from build123d import *

# Parameters (mm, degrees)
SKETCH1_R           = 2.1
SKETCH1_R_2         = 2.55
SKETCH1_R_3         = 2.54
BOSS_EXTRUDE1_DEPTH = 4


with BuildPart() as part:
    # Sketch1 → Boss-Extrude1 (new body)
    with BuildSketch(Plane(origin=(0, 0, 0), x_dir=(-1, 0, 0), z_dir=(0, 0, -1))):
        with BuildLine():
            Line((87.42535625, -29.106339063), (52.57464375, -20.393660937))
            ThreePointArc((52.57464375, -20.393660937), (47.11794562, -16.84635803), (45, -10.692235936))
            Line((45, -10.692235936), (45, -8))
            ThreePointArc((45, -8), (44.853553391, -7.646446609), (44.5, -7.5))
            Line((44.5, -7.5), (38, -7.5))
            ThreePointArc((38, -7.5), (37.646446609, -7.353553391), (37.5, -7))
            Line((37.5, -7), (37.5, 3))
            ThreePointArc((37.5, 3), (37.646446609, 3.353553391), (38, 3.5))
            Line((38, 3.5), (39.5, 3.5))
            ThreePointArc((39.5, 3.5), (39.853553391, 3.353553391), (40, 3))
            Line((40, 3), (40, -4.5))
            ThreePointArc((40, -4.5), (40.146446609, -4.853553391), (40.5, -5))
            Line((40.5, -5), (44.5, -5))
            ThreePointArc((44.5, -5), (44.853553391, -4.853553391), (45, -4.5))
            Line((45, -4.5), (45, 38.692235936))
            ThreePointArc((45, 38.692235936), (47.11794562, 44.84635803), (52.57464375, 48.393660937))
            Line((52.57464375, 48.393660937), (87.42535625, 57.106339063))
            ThreePointArc((87.42535625, 57.106339063), (92.88205438, 60.65364197), (95, 66.807764064))
            Line((95, 66.807764064), (95, 85))
            ThreePointArc((95, 85), (92.071067812, 92.071067812), (85, 95))
            Line((85, 95), (80.600023778, 95))
            ThreePointArc((80.600023778, 95), (75.38177505, 94.307249421), (70.525020806, 92.276988022))
            ThreePointArc((70.525020806, 92.276988022), (0, 73.215904175), (-70.525020806, 92.276988022))
            ThreePointArc((-70.525020806, 92.276988022), (-75.38177505, 94.307249421), (-80.600023778, 95))
            Line((-80.600023778, 95), (-85, 95))
            ThreePointArc((-85, 95), (-92.071067812, 92.071067812), (-95, 85))
            Line((-95, 85), (-95, 57.30993956))
            ThreePointArc((-95, 57.30993956), (-93.292887614, 51.721736358), (-88.754396995, 48.041471336))
            Line((-88.754396995, 48.041471336), (-51.245603005, 32.847708996))
            ThreePointArc((-51.245603005, 32.847708996), (-46.707112386, 29.167443975), (-45, 23.579240773))
            Line((-45, 23.579240773), (-45, -4.5))
            ThreePointArc((-45, -4.5), (-44.853553391, -4.853553391), (-44.5, -5))
            Line((-44.5, -5), (-40.5, -5))
            ThreePointArc((-40.5, -5), (-40.146446609, -4.853553391), (-40, -4.5))
            Line((-40, -4.5), (-40, 3))
            ThreePointArc((-40, 3), (-39.853553391, 3.353553391), (-39.5, 3.5))
            Line((-39.5, 3.5), (-38, 3.5))
            ThreePointArc((-38, 3.5), (-37.646446609, 3.353553391), (-37.5, 3))
            Line((-37.5, 3), (-37.5, -7))
            ThreePointArc((-37.5, -7), (-37.646446609, -7.353553391), (-38, -7.5))
            Line((-38, -7.5), (-44.5, -7.5))
            ThreePointArc((-44.5, -7.5), (-44.853553391, -7.646446609), (-45, -8))
            Line((-45, -8), (-45, -23.579240773))
            ThreePointArc((-45, -23.579240773), (-46.707112386, -29.167443975), (-51.245603005, -32.847708996))
            Line((-51.245603005, -32.847708996), (-88.754396995, -48.041471336))
            ThreePointArc((-88.754396995, -48.041471336), (-93.292887614, -51.721736358), (-95, -57.30993956))
            Line((-95, -57.30993956), (-95, -85))
            ThreePointArc((-95, -85), (-92.071067812, -92.071067812), (-85, -95))
            Line((-85, -95), (-80.600023778, -95))
            ThreePointArc((-80.600023778, -95), (-75.38177505, -94.307249421), (-70.525020806, -92.276988022))
            ThreePointArc((-70.525020806, -92.276988022), (0, -73.215904175), (70.525020806, -92.276988022))
            ThreePointArc((70.525020806, -92.276988022), (75.38177505, -94.307249421), (80.600023778, -95))
            Line((80.600023778, -95), (85, -95))
            ThreePointArc((85, -95), (92.071067812, -92.071067812), (95, -85))
            Line((95, -85), (95, -38.807764064))
            ThreePointArc((95, -38.807764064), (92.88205438, -32.65364197), (87.42535625, -29.106339063))
        make_face()
        with Locations(Location((-85, -85, 0), (0, 0, 180))):
            Circle(SKETCH1_R, mode=Mode.SUBTRACT)
        with Locations(Location((-85, 85, 0), (0, 0, 180))):
            Circle(SKETCH1_R, mode=Mode.SUBTRACT)
        with Locations(Location((85, 85, 0), (0, 0, 180))):
            Circle(SKETCH1_R, mode=Mode.SUBTRACT)
        with Locations(Location((85, -85, 0), (0, 0, 180))):
            Circle(SKETCH1_R, mode=Mode.SUBTRACT)
        with Locations(Location((25, 17.873209062, 0), (0, 0, 180))):
            Circle(SKETCH1_R_2, mode=Mode.SUBTRACT)
        with Locations(Location((25, -26.606790938, 0), (0, 0, 180))):
            Circle(SKETCH1_R_3, mode=Mode.SUBTRACT)
        with Locations(Location((-25, -26.606790938, 0), (0, 0, 180))):
            Circle(SKETCH1_R_3, mode=Mode.SUBTRACT)
        with Locations(Location((-25, 17.873209062, 0), (0, 0, 180))):
            Circle(SKETCH1_R_2, mode=Mode.SUBTRACT)
    extrude(amount=-BOSS_EXTRUDE1_DEPTH)


solid = part.part
Model file for the job. Use its own axes, mm. A direction names the side the tool comes from. Give positions to 0.01 mm unless a question says otherwise; leave off trailing zeros. Loops run counter-clockwise (first coordinate to the right, second up) from the corner with the lowest first, then second, coordinate; pieces in that order, holes last. Notation, with made-up numbers: (64, 84.25) - (72, 84.25) arc R19 cw to (72, 101.25) - close; hole circle Ø1 at (-10, 44.5). An arc over 180 degrees is marked (long way). Use one line per item in the form item = value.
(1) 3-axis set-ups, long thin cutter, end or side, ignore diameter. For faces 4 (the face through (46.66, -29.1, 1.97)), 5 (the face through (91.99, 92.15, 1.97)), 6 (the face through (-92.94, -32.73, 1.97)): which of +Z, -Z, +X, -X, +Y, -Y reach the whole face in a straight line?
Determined:
face_4 = +Z, -Z, +X
face_5 = +Z, -Z, +X, +Y
face_6 = +Z, -Z, -X
(2) Drill centre lines: L1, parallel to Y at x = 25, z = 1; L2, parallel to Y at x = 85, z = 2.5; L3, parallel to X at y = 85, z = 2. Where is each one in solid material? Low to high.
Determined:
L1 = -75.47 to -29.15, -24.07 to 15.32, 20.42 to 75.47
L2 = -95 to -87.1, -82.9 to -46.52, 46.52 to 82.9, 87.1 to 95
L3 = -95 to -87.1, -82.9 to -56.22, 56.22 to 82.9, 87.1 to 95
(3) Cut at A-A (x = -73). Give the cut face in (y, z).
Determined:
outline = (-93.5, 0) - (-25.5, 0) - (-25.5, 4) - (-93.5, 4) - close; (53.5, 0) - (93.5, 0) - (93.5, 4) - (53.5, 4) - close
(4) Cut at B-B (x = 25). Give the cut face in (y, z).
Determined:
outline = (-75.47, 0) - (-29.15, 0) - (-29.15, 4) - (-75.47, 4) - close; (-24.07, 0) - (15.32, 0) - (15.32, 4) - (-24.07, 4) - close; (20.42, 0) - (75.47, 0) - (75.47, 4) - (20.42, 4) - close
(5) Pull direction X, two halves, no side cores. Call faces 1 (the face through (1, 1, 4)), 2 (the face through (46.754, 29.236, 1.972)), 3 (the face through (-26.88, 16.15, 1.97)): pulls with the +X half, pulls with the -X half, needs draft (parallel to the pull), parting line crosses it, or undercut.
Determined:
face_1 = needs draft
face_2 = pulls with the +X half
face_3 = undercut
(6) Cut at D-D (z = 0.95). Count the separate pieces of the cut face and the enclosed holes in it, then the cut area to 3 significant figures.
Determined:
separate_pieces = 1
enclosed_holes = 8
area = 23,400 mm^2
(7) Cut at C-C (y = 9). Give the cut face in (x, z).
Determined:
outline = (-45, 0) - (45, 0) - (45, 4) - (-45, 4) - close
(8) Drop flat-ended pins along their axis: P1, Ø3, axis at x = 46, y = 9, coming from the -Z side; P2, Ø4.5, axis at x = -25, y = 17.87, coming from the -Z side; P3, Ø1.2, axis at y = 13, z = 2.5, coming from the +X side; P4, Ø1.2, axis at x = -39, z = 2, coming from the -Y side. Give the stop position or say it passes through.
Determined:
P1 = 0
P2 = through
P3 = 45
P4 = -78.93
